from build123d import *

# Parameters (mm, degrees)
BOSS_EXTRUDE1_DEPTH = 23
CUT_EXTRUDE1_DEPTH  = 3


with BuildPart() as part:
    # Sketch1 → Revolve1 (revolve)
    with BuildSketch(Plane.XY):
        Polygon((-57.5, 0), (-57.5, -7.939339828), (-56.439339828, -9), (56.439339828, -9), (57.5, -7.939339828), (57.5, 0), align=None)
    revolve(axis=Axis((-100, 0, 0), (1, 0, 0)))

    # Sketch2 → Boss-Extrude1 (add)
    with BuildSketch(Plane.ZY.offset(41.5)):
        with BuildLine():
            ThreePointArc((-7.947510586, 8.990944082), (-10.426372404, 11.920385617), (-10.622991997, 15.752842316))
            ThreePointArc((-10.622991997, 15.752842316), (-10.272175532, 15.983817124), (-9.91633903, 16.206980602))
            ThreePointArc((-9.91633903, 16.206980602), (-6.511892526, 14.43606908), (-4.876935192, 10.964283065))
            ThreePointArc((-4.876935192, 10.964283065), (-3.380790682, 11.513915683), (-1.825, 11.860412092))
            ThreePointArc((-1.825, 11.860412092), (-2.326575595, 15.664989012), (-0.42, 18.995357328))
            ThreePointArc((-0.42, 18.995357328), (0, 19), (0.42, 18.995357328))
            ThreePointArc((0.42, 18.995357328), (2.326575595, 15.664989012), (1.825, 11.860412092))
            ThreePointArc((1.825, 11.860412092), (3.380790682, 11.513915683), (4.876935192, 10.964283065))
            ThreePointArc((4.876935192, 10.964283065), (6.511892526, 14.43606908), (9.91633903, 16.206980602))
            ThreePointArc((9.91633903, 16.206980602), (10.272175532, 15.983817124), (10.622991997, 15.752842316))
            ThreePointArc((10.622991997, 15.752842316), (10.426372404, 11.920385617), (7.947510586, 8.990944082))
            ThreePointArc((7.947510586, 8.990944082), (9.068994892, 7.858328807), (10.030477919, 6.587071635))
            ThreePointArc((10.030477919, 6.587071635), (13.282880781, 8.623799215), (17.104310483, 8.273002049))
            ThreePointArc((17.104310483, 8.273002049), (17.283007912, 7.892885247), (17.453259094, 7.508911173))
            ThreePointArc((17.453259094, 7.508911173), (15.215869643, 4.391144013), (11.546742716, 3.266914852))
            ThreePointArc((11.546742716, 3.266914852), (11.877857303, 1.707778059), (11.999414778, 0.118511503))
            ThreePointArc((11.999414778, 0.118511503), (15.836648241, 0.073534032), (18.861784211, -2.2875962))
            ThreePointArc((18.861784211, -2.2875962), (18.806607396, -2.703981927), (18.742239747, -3.119046212))
            ThreePointArc((18.742239747, -3.119046212), (15.174435781, -4.532254788), (11.479965619, -3.49433676))
            ThreePointArc((11.479965619, -3.49433676), (10.915583944, -4.984980156), (10.15862223, -6.387675194))
            ThreePointArc((10.15862223, -6.387675194), (13.36239178, -8.500077686), (14.630774723, -12.12189882))
            ThreePointArc((14.630774723, -12.12189882), (14.359241913, -12.442353945), (14.080691707, -12.756728462))
            ThreePointArc((14.080691707, -12.756728462), (10.315225776, -12.016694717), (7.768380551, -9.146161141))
            ThreePointArc((7.768380551, -9.146161141), (6.487689809, -10.095042394), (5.092538901, -10.865820151))
            ThreePointArc((5.092538901, -10.865820151), (6.645670343, -14.374974798), (5.754597637, -18.107584213))
            ThreePointArc((5.754597637, -18.107584213), (5.35291858, -18.230366499), (4.948623539, -18.344239561))
            ThreePointArc((4.948623539, -18.344239561), (2.181004471, -15.68591898), (1.590389547, -11.894143983))
            ThreePointArc((1.590389547, -11.894143983), (0, -12), (-1.590389547, -11.894143983))
            ThreePointArc((-1.590389547, -11.894143983), (-2.181004471, -15.68591898), (-4.948623539, -18.344239561))
            ThreePointArc((-4.948623539, -18.344239561), (-5.35291858, -18.230366499), (-5.754597637, -18.107584213))
            ThreePointArc((-5.754597637, -18.107584213), (-6.645670343, -14.374974798), (-5.092538901, -10.865820151))
            ThreePointArc((-5.092538901, -10.865820151), (-6.487689809, -10.095042394), (-7.768380551, -9.146161141))
            ThreePointArc((-7.768380551, -9.146161141), (-10.315225776, -12.016694717), (-14.080691707, -12.756728462))
            ThreePointArc((-14.080691707, -12.756728462), (-14.359241913, -12.442353945), (-14.630774723, -12.12189882))
            ThreePointArc((-14.630774723, -12.12189882), (-13.36239178, -8.500077686), (-10.15862223, -6.387675194))
            ThreePointArc((-10.15862223, -6.387675194), (-10.915583944, -4.984980156), (-11.479965619, -3.49433676))
            ThreePointArc((-11.479965619, -3.49433676), (-15.174435781, -4.532254788), (-18.742239747, -3.119046212))
            ThreePointArc((-18.742239747, -3.119046212), (-18.806607396, -2.703981927), (-18.861784211, -2.2875962))
            ThreePointArc((-18.861784211, -2.2875962), (-15.836648241, 0.073534032), (-11.999414778, 0.118511503))
            ThreePointArc((-11.999414778, 0.118511503), (-11.877857303, 1.707778059), (-11.546742716, 3.266914852))
            ThreePointArc((-11.546742716, 3.266914852), (-15.215869643, 4.391144013), (-17.453259094, 7.508911173))
            ThreePointArc((-17.453259094, 7.508911173), (-17.283007912, 7.892885247), (-17.104310483, 8.273002049))
            ThreePointArc((-17.104310483, 8.273002049), (-13.282880781, 8.623799215), (-10.030477919, 6.587071635))
            ThreePointArc((-10.030477919, 6.587071635), (-9.068994892, 7.858328807), (-7.947510586, 8.990944082))
        make_face()
    extrude(amount=-BOSS_EXTRUDE1_DEPTH)

    # Sketch4 → Cut-Extrude1 (cut)
    with BuildSketch(Plane(origin=(0, 9, 0), x_dir=(1, 0, 0), z_dir=(0, 1, 0))):
        with BuildLine():
            Line((33.550041919, 3), (51.550041919, 3))
            ThreePointArc((51.550041919, 3), (54.550041919, 0), (51.550041919, -3))
            Line((51.550041919, -3), (33.550041919, -3))
            ThreePointArc((33.550041919, -3), (30.550041919, 0), (33.550041919, 3))
        make_face()
    extrude(amount=-CUT_EXTRUDE1_DEPTH, mode=Mode.SUBTRACT)


solid = part.part
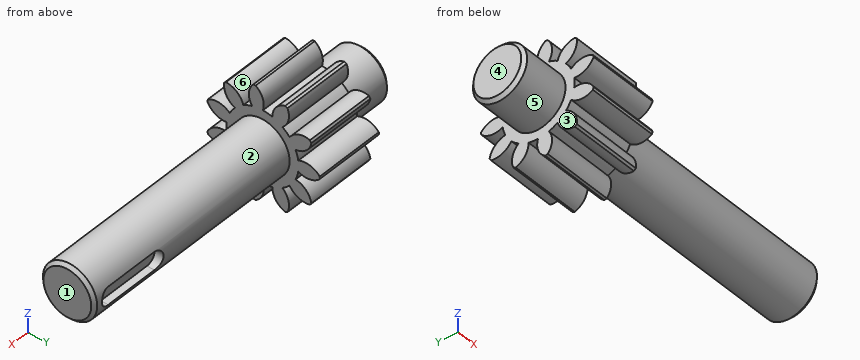
Input: part model. Units: mm. Frame: model coordinates. Face numbers are marked on the shaded views. A direction names the side the tool comes from. Coordinates: 2 decimals unless noted, no trailing zeros. Loops run counter-clockwise (first coordinate to the right, second up) from the corner with the lowest first, then second, coordinate; pieces in that order, holes last.
(1) Section C-C on x = 25.5. Return the cut outline in (y, z), then the cut area to 3 significant figures.
(2) Section B-B on x = 44. Return the cut outline in (y, z), then the cut area to 3 significant figures.
(3) Material intervals for probe 1 along Y at (x, z) = (-31, -12.5); probe 2 along X at (y, z) = (-13, -2); probe 3 along Z at (x, y) = (49.5, 8), sorted ascending.
(4) First-contact query: pin 1 Ø2 at (x, y) = (38.5, 7) entering from +Z; pin 2 Ø3 at (x, y) = (45.5, 5.5) entering from +Z; pin 3 Ø5 at (y, z) = (3, -12.5) entering from +X; pin 4 Ø12 at (x, z) = (-39.5, 4.5) entering from -Y. Flat tips, straight axial feed; report the tip coordinate or a pass-through.
(5) Set-up query: the marked faces 1, 2 and 3. Return all of +Z, -Z, +X, -X, +Y, -Y with unobstructed straight access to the full face (end or side cutting, diameter ignored); none if empty.
(6) Section A-A on y = -15.5. Return the cut outline in (x, z), then the cut area to 4 significant figures.
(7) Pull-direction query (Y, two-part tool) for the marked faces 4, 5 and 6; classes: released by +Y, released by -Y, zero draft, split by the parting line, or undercut.
Data:
1. outline: circle Ø18 at (0, 0)
1. area: 254 mm2
2. outline: (6, -3) - (6, 3) - (8.49, 3) arc R9 ccw (long way) to (8.49, -3) - close
2. area: 237 mm2
3. probe 1: y = -12.76 to -7.6, -4.05 to 0.26, 3.32 to 8.38
3. probe 2: x = -41.5 to -18.5
3. probe 3: z = -4.12 to -3, 3 to 4.12
4. pin 1: stops at z = 6.71
4. pin 2: stops at z = 8.06
4. pin 3: stops at x = -18.5
4. pin 4: stops at y = -18.34
5. face 1: +Z, -Z, +X, +Y, -Y
5. face 2: +X
5. face 3: -X
6. outline: (-41.5, -6.64) - (-18.5, -6.64) - (-18.5, -2.09) - (-41.5, -2.09) - close; (-41.5, 2.09) - (-18.5, 2.09) - (-18.5, 6.64) - (-41.5, 6.64) - close
6. area: 209.5 mm2
7. face 4: zero draft
7. face 5: split by the parting line
7. face 6: undercut
